from build123d import *

# Parameters (mm, degrees)
SKETCH1_W           = 30
SKETCH1_H           = 45
SKETCH1_R           = 3
BOSS_EXTRUDE1_DEPTH = 5
SKETCH2_W           = 30
SKETCH2_H           = 5
BOSS_EXTRUDE2_DEPTH = 30
SKETCH3_R           = 4
CUT_EXTRUDE1_DEPTH  = 30
FILLET1_R           = 5


with BuildPart() as part:
    # Sketch1 → Boss-Extrude1 (new body)
    with BuildSketch(Plane.XY):
        with Locations((15, 22.5)):
            Rectangle(SKETCH1_W, SKETCH1_H)
        with Locations((15, 30)):
            Circle(SKETCH1_R, mode=Mode.SUBTRACT)
    extrude(amount=BOSS_EXTRUDE1_DEPTH)

    # Sketch2 → Boss-Extrude2 (add)
    with BuildSketch(Plane.XY.offset(5)):
        with Locations((15, 2.5)):
            Rectangle(SKETCH2_W, SKETCH2_H)
    extrude(amount=BOSS_EXTRUDE2_DEPTH)

    # Sketch3 → Cut-Extrude1 (cut)
    with BuildSketch(Plane(origin=(0, 5, 0), x_dir=(1, 0, 0), z_dir=(0, 1, 0))):
        with Locations(Location((15, -20, 0), (0, 0, 270))):
            Circle(SKETCH3_R)
    extrude(amount=-CUT_EXTRUDE1_DEPTH, mode=Mode.SUBTRACT)

    # Fillet1
    fillet1_edges = [part.edges().sort_by_distance(p)[0] for p in [
        (15, 5, 5),
        (0, 2.5, 35),
        (30, 2.5, 35),
        (15, 0, 0),
        (0, 45, 2.5),
        (30, 45, 2.5),
    ]]
    fillet(fillet1_edges, radius=FILLET1_R)


solid = part.part
For this review, take the finished solid that the model builds, in its own axes (mm). A direction names the side the tool comes from. Coordinates: 2 decimals unless noted, no trailing zeros. Write each loop counter-clockwise with the first axis right and the second up, starting at its lowest first coordinate (ties: lowest second). Pieces come first, ordered by that corner, then holes. Notation, with made-up numbers: (69.25, 35) -> (86.25, 35) arc R16 ccw to (86.25, 63) -> close; hole circle Ø11 at (-1, -11.75). An arc over 180 degrees is marked (long way). Write each question's results on one line, items separated by ' | '. Start each with the question number.
1) Insertion check: pin 1 (7.5 mm diameter, centred on x = 8.5, z = 19, fed in from +Y); pin 2 (1.5 mm diameter, centred on x = 9.5, y = 23, fed in from +Z). Each pin has a flat end and moves straight along its axis. Give the tip position at first contact, or say it passes through.
2) For faces 1 (the face through (11, 28, 5)), 2 (the face through (1, 43, 3)), list the 3-axis set-ups (+Z, -Z, +X, -X, +Y, -Y) from which the entire face can be reached by the end or side of a thin tool; tool diameter is ignored.
3) Consider section C-C (x = 15). Write out the cut boundary in (y, z).
4) Wall thickness on L1, parallel to X at y = 1, z = 20; L2, parallel to Y at x = 24, z = 18: over which ranges is each line inside the solid? List them lowest first. Write a range as [from, to].
5) Consider section A-A (z = 20). Write out the cut boundary in (x, y), plus the area to 3 significant figures.
6) Consider section D-D (x = 21.5). Write out the cut boundary in (y, z).
7) The part is to be moulded in two halves that separate along X. For faces 3 (the face through (15, 45, 2)), 4 (the face through (28, 3, 34)), 5 (the face through (18.966, 2.535, 19.479)), say which applies: +X half, -X half, draft (parallel to the pull), parting line (faces both ways), or undercut.
8) Consider section B-B (y = 30). Write out the cut boundary in (x, z), plus the area to 3 significant figures.
Geometry says:
1) pin 1: y = 5 | pin 2: z = 5
2) face 1: +Z, +X, -X, +Y | face 2: +Z, -Z, -X, +Y
3) outline: (0, 5) arc R5 ccw to (5, 0) -> (27, 0) -> (27, 5) -> (10, 5) arc R5 cw to (5, 10) -> (5, 16) -> (0, 16) -> close; (0, 24) -> (5, 24) -> (5, 35) -> (0, 35) -> close; (33, 0) -> (45, 0) -> (45, 5) -> (33, 5) -> close
4) L1: [0, 11], [19, 30] | L2: [0, 5]
5) outline: (0, 0) -> (11, 0) -> (11, 5) -> (0, 5) -> close; (19, 0) -> (30, 0) -> (30, 5) -> (19, 5) -> close | area: 110 mm^2
6) outline: (0, 5) arc R5 ccw to (5, 0) -> (45, 0) -> (45, 5) -> (10, 5) arc R5 cw to (5, 10) -> (5, 35) -> (0, 35) -> close
7) face 3: draft | face 4: +X half | face 5: undercut
8) outline: (0, 0) -> (12, 0) -> (12, 5) -> (0, 5) -> close; (18, 0) -> (30, 0) -> (30, 5) -> (18, 5) -> close | area: 120 mm^2
